from build123d import *

# Parameters (mm, degrees)
F1_DEPTH = 1.27
F2_DEPTH = 1.27
F3_R     = 0.508
F4_R     = 0.508
F5_DEPTH = 25.4


with BuildPart() as f1:
    # F0 (on Front) → F1 (new body, symmetric)
    with BuildSketch(Plane.XZ):
        with BuildLine():
            ThreePointArc((1.6980241155, -2.3923439956), (0, -2.9337), (-1.6980241155, -2.3923439956))
            Line((-1.6980241155, -2.3923439956), (-2.906111014, -50.7841772133))
            ThreePointArc((-2.906111014, -50.7841772133), (0, -49.6643153071), (2.906111014, -50.7841772133))
            Line((2.906111014, -50.7841772133), (1.6980241155, -2.3923439956))
        make_face()
        with BuildLine():
            ThreePointArc((1.6980241155, -2.3923439956), (2.6065388006, -1.3463102061), (2.9337, 0))
            ThreePointArc((2.9337, 0), (-1.3463102061, 2.6065388006), (-1.6980241155, -2.3923439956))
            Line((-1.6980241155, -2.3923439956), (-1.6383, 0))
            ThreePointArc((-1.6383, 0), (0, 1.6383), (1.6383, 0))
            Line((1.6383, 0), (1.6980241155, -2.3923439956))
        make_face()
        with BuildLine():
            Line((-1.6383, 0), (-1.6980241155, -2.3923439956))
            ThreePointArc((-1.6980241155, -2.3923439956), (0, -2.9337), (1.6980241155, -2.3923439956))
            Line((1.6980241155, -2.3923439956), (1.6383, 0))
            ThreePointArc((1.6383, 0), (0, -1.6383), (-1.6383, 0))
        make_face()
        with BuildLine():
            ThreePointArc((2.906111014, -50.7841772133), (0, -49.6643153071), (-2.906111014, -50.7841772133))
            ThreePointArc((-2.906111014, -50.7841772133), (-3.273195149, -51.1593220926), (-3.5922005773, -51.5761193807))
            Line((-3.5922005773, -51.5761193807), (-3.5922005773, -53.9950153071))
            Line((-3.5922005773, -53.9950153071), (-2.7051, -53.9950153071))
            ThreePointArc((-2.7051, -53.9950153071), (0, -51.2899153071), (2.7051, -53.9950153071))
            Line((2.7051, -53.9950153071), (3.5922005773, -53.9950153071))
            Line((3.5922005773, -53.9950153071), (3.5922005773, -51.5761193807))
            ThreePointArc((3.5922005773, -51.5761193807), (3.273195149, -51.1593220926), (2.906111014, -50.7841772133))
        make_face()
        with BuildLine():
            ThreePointArc((4.3307, -53.9950153071), (4.1419624292, -52.7304562041), (3.5922005773, -51.5761193807))
            Line((3.5922005773, -51.5761193807), (3.5922005773, -53.9950153071))
            Line((3.5922005773, -53.9950153071), (4.3307, -53.9950153071))
        make_face()
        with BuildLine():
            Line((3.5922005773, -51.5533201396), (3.5922005773, -51.5761193807))
            ThreePointArc((3.5922005773, -51.5761193807), (4.1419624292, -52.7304562041), (4.3307, -53.9950153071))
            Line((4.3307, -53.9950153071), (5.4972005773, -53.9950153071))
            Line((5.4972005773, -53.9950153071), (5.4972005773, -51.5533201396))
            Line((5.4972005773, -51.5533201396), (3.5922005773, -51.5533201396))
        make_face()
        with BuildLine():
            Line((-3.5922005773, -53.9950153071), (-3.5922005773, -51.5761193807))
            ThreePointArc((-3.5922005773, -51.5761193807), (-4.1419624292, -52.7304562041), (-4.3307, -53.9950153071))
            Line((-4.3307, -53.9950153071), (-3.5922005773, -53.9950153071))
        make_face()
        with BuildLine():
            ThreePointArc((-4.3307, -53.9950153071), (-4.1419624292, -52.7304562041), (-3.5922005773, -51.5761193807))
            Line((-3.5922005773, -51.5761193807), (-3.5922005773, -51.5533201396))
            Line((-3.5922005773, -51.5533201396), (-5.4972005773, -51.5533201396))
            Line((-5.4972005773, -51.5533201396), (-5.4972005773, -53.9950153071))
            Line((-5.4972005773, -53.9950153071), (-4.3307, -53.9950153071))
        make_face()
    extrude(amount=F1_DEPTH, both=True)

    # F0 (on Front) → F2 (join, symmetric)
    with BuildSketch(Plane.XZ):
        with BuildLine():
            ThreePointArc((1.6980241155, -2.3923439956), (0, -2.9337), (-1.6980241155, -2.3923439956))
            Line((-1.6980241155, -2.3923439956), (-2.906111014, -50.7841772133))
            ThreePointArc((-2.906111014, -50.7841772133), (0, -49.6643153071), (2.906111014, -50.7841772133))
            Line((2.906111014, -50.7841772133), (1.6980241155, -2.3923439956))
        make_face()
        with BuildLine():
            ThreePointArc((1.6980241155, -2.3923439956), (2.6065388006, -1.3463102061), (2.9337, 0))
            ThreePointArc((2.9337, 0), (-1.3463102061, 2.6065388006), (-1.6980241155, -2.3923439956))
            Line((-1.6980241155, -2.3923439956), (-1.6383, 0))
            ThreePointArc((-1.6383, 0), (0, 1.6383), (1.6383, 0))
            Line((1.6383, 0), (1.6980241155, -2.3923439956))
        make_face()
        with BuildLine():
            Line((-1.6383, 0), (-1.6980241155, -2.3923439956))
            ThreePointArc((-1.6980241155, -2.3923439956), (0, -2.9337), (1.6980241155, -2.3923439956))
            Line((1.6980241155, -2.3923439956), (1.6383, 0))
            ThreePointArc((1.6383, 0), (0, -1.6383), (-1.6383, 0))
        make_face()
        with BuildLine():
            ThreePointArc((2.906111014, -50.7841772133), (0, -49.6643153071), (-2.906111014, -50.7841772133))
            ThreePointArc((-2.906111014, -50.7841772133), (-3.273195149, -51.1593220926), (-3.5922005773, -51.5761193807))
            Line((-3.5922005773, -51.5761193807), (-3.5922005773, -53.9950153071))
            Line((-3.5922005773, -53.9950153071), (-2.7051, -53.9950153071))
            ThreePointArc((-2.7051, -53.9950153071), (0, -51.2899153071), (2.7051, -53.9950153071))
            Line((2.7051, -53.9950153071), (3.5922005773, -53.9950153071))
            Line((3.5922005773, -53.9950153071), (3.5922005773, -51.5761193807))
            ThreePointArc((3.5922005773, -51.5761193807), (3.273195149, -51.1593220926), (2.906111014, -50.7841772133))
        make_face()
    extrude(amount=F2_DEPTH, both=True)

    # F3 (on face) + F4 (on face) → F5 (cut)
    with BuildSketch(Plane.XY.offset(-51.5533201396)):
        with Locations((-4.5447005773, 0)):
            Circle(F3_R)
    with BuildSketch(Plane.XY.offset(-51.5533201396)):
        with Locations((4.5447005773, 0)):
            Circle(F4_R)
    extrude(amount=-F5_DEPTH, mode=Mode.SUBTRACT)


solid = f1.part
The model under review builds one solid part; all positions refer to its coordinate system, in mm. A direction names the side the tool comes from. Coordinates: 2 decimals unless noted, no trailing zeros. Write each loop counter-clockwise with the first axis right and the second up, starting at its lowest first coordinate (ties: lowest second). Pieces come first, ordered by that corner, then holes. Notation, with made-up numbers: M 86,56.5 L 117,56.5 A25 cw 117,90.5 Z; hole C 6,-7.75 d3. An arc over 180 degrees is marked long. Put each result on its own line as item: value.
1) For faces 4 (the flat face through (5.497, 0, -53)), 5 (the flat face through (-5, -1, -51.553)), 6 (the flat face through (5, -1, -51.553)), list the 3-axis set-ups (+Z, -Z, +X, -X, +Y, -Y) from which the entire face can be reached by the end or side of a thin tool; tool diameter is ignored.
Computed:
face 4: +Z, -Z, +X, +Y, -Y
face 5: +Z, -X, +Y, -Y
face 6: +Z, +X, +Y, -Y
2) Add section A-A on x = 0. Give the boundary of the cut face in (y, z), then the cut area to 3 significant figures.
Computed:
outline: M -1.27,-51.29 L 1.27,-51.29 L 1.27,-1.64 L -1.27,-1.64 Z; M -1.27,1.64 L 1.27,1.64 L 1.27,2.93 L -1.27,2.93 Z
area: 129 mm2
3) Wall thickness on probe 1 along Z at (x, y) = (0, -0.2); probe 2 along Z at (x, y) = (-4, 0); probe 3 along Z at (x, y) = (-1.5, 0.7): over which ranges is each line inside the solid? List them lowest first. Write a range as [from, to].
Computed:
probe 1: z = [-51.29, -1.64], [1.64, 2.93]
probe 2: z = [-54, -51.55]
probe 3: z = [-51.74, -0.66], [0.66, 2.52]
4) Add section B-B on y = 0. State how many separate pieces and enclosed holes the cut face has, then the cut area to 3 significant figures.
Computed:
separate pieces: 3
enclosed holes: 1
area: 256 mm2
5) Clearance check with flat-ended pins moving along their axes: pin 1 Ø3 at (x, z) = (0, 0) entering from -Y; pin 2 Ø1.5 at (x, y) = (-1.5, -0.5) entering from +Z; pin 3 Ø1.2 at (x, y) = (-4.54, 0) entering from +Z; pin 4 Ø1 at (x, y) = (-1.5, 0.5) entering from -Z. State where each tip first meets the part, or that it passes through.
Computed:
pin 1: passes through
pin 2: stops at z = 2.84
pin 3: stops at z = -51.55
pin 4: stops at z = -52.17
6) Add section C-C on z = -26.5. Give the boundary of the cut face in (x, y), then the cut area to 3 significant figures.
Computed:
outline: M -2.3,-1.27 L 2.3,-1.27 L 2.3,1.27 L -2.3,1.27 Z
area: 11.7 mm2
7) Draft analysis for pull direction Z (two halves, no side actions). For faces 1 (the flat face through (-5.497, 0, -53)), 2 (the cylindrical face through (0.213, -0.018, 1.624)), 3 (the flat face through (-3.8, 0, -53.995)), state which applies: released by +Z, released by -Z, zero draft, split by the parting line, or undercut.
Computed:
face 1: zero draft
face 2: undercut
face 3: released by -Z
